```python
from build123d import *

# Parameters (mm, degrees)
EXTRUDE_1_DEPTH     = 2.2
EXTRUDE_1_2_DEPTH   = 2.2
SKETCH_1_3_W        = 12.8
SKETCH_1_3_H        = 18.7
SKETCH_1_3_R        = 1.25
EXTRUDE_2_DEPTH     = 7
SKETCH_1_4_R        = 2.5
SKETCH_1_4_R_2      = 1.25
CUT_EXTRUDE_1_DEPTH = 2.2
FILLET_1_R          = 2


with BuildPart() as part:
    # Sketch 1 → Extrude 1 (new body)
    with BuildSketch(Plane(origin=(0, 0, 0), x_dir=(1, 0, 0), z_dir=(0, 1, 0))):
        with BuildLine():
            Line((-6.4, 9.35), (-8.35, 9.35))
            ThreePointArc((-8.35, 9.35), (-9.057106781, 9.057106781), (-9.35, 8.35))
            Line((-9.35, 8.35), (-9.35, -8.35))
            ThreePointArc((-9.35, -8.35), (-9.057106781, -9.057106781), (-8.35, -9.35))
            Line((-8.35, -9.35), (-6.4, -9.35))
            Line((-6.4, -9.35), (-6.4, 9.35))
        make_face()
    extrude(amount=EXTRUDE_1_DEPTH)



with BuildPart() as body_2:
    # Sketch 1 → Extrude 1 2 (new body)
    with BuildSketch(Plane(origin=(0, 0, 0), x_dir=(1, 0, 0), z_dir=(0, 1, 0))):
        with BuildLine():
            Line((8.35, 9.35), (6.4, 9.35))
            Line((6.4, 9.35), (6.4, -9.35))
            Line((6.4, -9.35), (8.35, -9.35))
            ThreePointArc((8.35, -9.35), (9.057106781, -9.057106781), (9.35, -8.35))
            Line((9.35, -8.35), (9.35, 8.35))
            ThreePointArc((9.35, 8.35), (9.057106781, 9.057106781), (8.35, 9.35))
        make_face()
    extrude(amount=EXTRUDE_1_2_DEPTH)


with BuildPart() as part_1:
    add(part.part)

    add(body_2.part)  # Extrude 2 merges body 2
    # Sketch 1_3 → Extrude 2 (add)
    with BuildSketch(Plane(origin=(0, 0, 0), x_dir=(1, 0, 0), z_dir=(0, 1, 0))):
        Rectangle(SKETCH_1_3_W, SKETCH_1_3_H)
        with Locations(Location((0, 5, 0), (0, 0, 270))):
            Circle(SKETCH_1_3_R, mode=Mode.SUBTRACT)
        with Locations(Location((0, -5, 0), (0, 0, 270))):
            Circle(SKETCH_1_3_R, mode=Mode.SUBTRACT)
    extrude(amount=EXTRUDE_2_DEPTH)

    # Sketch 1_4 → Cut-Extrude 1 (cut)
    # profile 1 of 2: a face of its own
    with BuildSketch(Plane(origin=(0, 0, 0), x_dir=(1, 0, 0), z_dir=(0, 1, 0))):
        with Locations(Location((0, -5, 0), (0, 0, 270))):
            Circle(SKETCH_1_4_R)
        with Locations(Location((0, -5, 0), (0, 0, 270))):
            Circle(SKETCH_1_4_R_2, mode=Mode.SUBTRACT)
    # profile 2 of 2: a face of its own
    with BuildSketch(Plane(origin=(0, 0, 0), x_dir=(1, 0, 0), z_dir=(0, 1, 0))):
        with Locations(Location((0, 5, 0), (0, 0, 270))):
            Circle(SKETCH_1_4_R)
        with Locations(Location((0, 5, 0), (0, 0, 270))):
            Circle(SKETCH_1_4_R_2, mode=Mode.SUBTRACT)
    extrude(amount=CUT_EXTRUDE_1_DEPTH, mode=Mode.SUBTRACT)

    # Fillet 1
    # the kernel refuses this fillet: 2 mm, written as the material it takes off along each edge
    with BuildSketch(Plane(origin=(0, 2.2, 5), x_dir=(0, 0, 1), z_dir=(-1, 0, 0))) as fillet_1_piece_1:
        with BuildLine():
            CenterArc((3.25, 1.854049622), FILLET_1_R, 180, 67.975687163)
            Line((2.5, 0), (2.485, -0.037080992))
            ThreePointArc((2.485, -0.037080992), (1.875, -0.04), (1.25, -0.04))
            Line((1.25, -0.04), (1.21, 0))
            Line((1.21, 0), (1.21, 1.854049622))
            Line((1.21, 1.854049622), (1.25, 1.854049622))
        make_face()
    revolve(axis=Axis((0, 2.2, 5), (0, 1, 0)), mode=Mode.SUBTRACT)
    with BuildSketch(Plane(origin=(0, 2.2, -5), x_dir=(0, 0, 1), z_dir=(-1, 0, 0))) as fillet_1_piece_2:
        with BuildLine():
            CenterArc((3.25, 1.854049622), FILLET_1_R, 180, 67.975687163)
            Line((2.5, 0), (2.485, -0.037080992))
            ThreePointArc((2.485, -0.037080992), (1.875, -0.04), (1.25, -0.04))
            Line((1.25, -0.04), (1.21, 0))
            Line((1.21, 0), (1.21, 1.854049622))
            Line((1.21, 1.854049622), (1.25, 1.854049622))
        make_face()
    revolve(axis=Axis((0, 2.2, -5), (0, 1, 0)), mode=Mode.SUBTRACT)


solid = part_1.part
```
Could you check a few things on this model? Use its own coordinates, in mm. A direction names the side the tool comes from. Round coordinates to 2 decimals unless told otherwise and drop trailing zeros. Loops run counter-clockwise (first coordinate to the right, second up) from the corner with the lowest first, then second, coordinate; pieces in that order, holes last. Notation, with made-up numbers: (70, -12) -> (105, -12) arc R20 cw to (105, 11) -> close; hole circle Ø3 at (41.25, 85). An arc over 180 degrees is marked (long way). One line per question, with ' | ' between items.
(1) Thinking about a two-plate mould opening in X: for faces 1 (the face through (0.05, 5.51, 3.75)), 2 (the face through (6.4, 5, 0)), 3 (the face through (-9.065, 1.085, 9.049)), which applies, released by +X, released by -X, zero draft, split by the parting line, or undercut?
Model answer:
face 1: undercut | face 2: released by +X | face 3: released by -X
(2) For faces 4 (the face through (8, 2.2, 0)), 5 (the face through (-8, 2.2, 0)), 6 (the face through (0.751, 1.085, 7.385)), which set-ups out of +Z, -Z, +X, -X, +Y, -Y let a thin tool reach every point of the face, with its end or its side?
Model answer:
face 4: +Z, -Z, +X, +Y | face 5: +Z, -Z, -X, +Y | face 6: -Y
(3) If we section it at A-A on z = 5: List the corners of the cut face in (x, y) for me, and give its area (3 significant figures).
Model answer:
outline: (-9.35, 0) -> (-2.5, 0) -> (-2.5, 2.2) arc R2 ccw to (-1.25, 4.05) -> (-1.25, 7) -> (-6.4, 7) -> (-6.4, 2.2) -> (-9.35, 2.2) -> close; (1.25, 4.05) arc R2 ccw to (2.5, 2.2) -> (2.5, 0) -> (9.35, 0) -> (9.35, 2.2) -> (6.4, 2.2) -> (6.4, 7) -> (1.25, 7) -> close | area: 78.3 mm^2
(4) If we section it at B-B on x = 0: List the corners of the cut face in (y, z) for me, and give its area (3 significant figures).
Model answer:
outline: (0, -9.35) -> (7, -9.35) -> (7, -6.25) -> (4.05, -6.25) arc R2 ccw to (2.2, -7.5) -> (0, -7.5) -> close; (0, -2.5) -> (2.2, -2.5) arc R2 ccw to (4.05, -3.75) -> (7, -3.75) -> (7, 3.75) -> (4.05, 3.75) arc R2 ccw to (2.2, 2.5) -> (0, 2.5) -> close; (0, 7.5) -> (2.2, 7.5) arc R2 ccw to (4.05, 6.25) -> (7, 6.25) -> (7, 9.35) -> (0, 9.35) -> close | area: 82.3 mm^2
(5) For pin 1 Ø2 at (y, z) = (4, 1.5) entering from +X; pin 2 Ø3 at (y, z) = (6, 3) entering from -X; pin 3 Ø2.5 at (x, z) = (8.5, 3) entering from +Y, each with a flat end and sliding along its axis, tell me the tip position at first contact or that it passes through.
Model answer:
pin 1: stops at x = 6.4 | pin 2: stops at x = -6.4 | pin 3: stops at y = 2.2
(6) If we section it at C-C on y = 5.5: List the corners of the cut face in (x, z) for me.
Model answer:
outline: (-6.4, -9.35) -> (6.4, -9.35) -> (6.4, 9.35) -> (-6.4, 9.35) -> close; hole circle Ø2.5 at (0, -5); hole circle Ø2.5 at (0, 5)
(7) If I drill on probe 1 along X at (y, z) = (5.5, -5); probe 2 along Z at (x, y) = (-2, 0.5); probe 3 along X at (y, z) = (5.75, -1.5), over which ranges is the centre line in solid material (lowest first)?
Model answer:
probe 1: x = -6.4 to -1.25, 1.25 to 6.4 | probe 2: z = -9.35 to -6.5, -3.5 to 3.5, 6.5 to 9.35 | probe 3: x = -6.4 to 6.4
(8) If we section it at D-D on z = 1.75: List the corners of the cut face in (x, y) for me.
Model answer:
outline: (-9.35, 0) -> (9.35, 0) -> (9.35, 2.2) -> (6.4, 2.2) -> (6.4, 7) -> (-6.4, 7) -> (-6.4, 2.2) -> (-9.35, 2.2) -> close
